Geometry: final body of the model. Coordinates: model frame, mm. A direction names the side the tool comes from. Give positions to 0.01 mm unless a question says otherwise; leave off trailing zeros. Loops run counter-clockwise (first coordinate to the right, second up) from the corner with the lowest first, then second, coordinate; pieces in that order, holes last. Notation, with made-up numbers: (64, -9.75) -> (95, -9.75) arc R16 ccw to (95, 6.25) -> close; hole circle Ø6 at (9, 68.5). An arc over 180 degrees is marked (long way). Answer in a Markdown table with one row per item. Add a question column.
1) Section query B-B (z = -25.5). Return the cut outline in (x, y).
2) Section query D-D (z = 6). Return the cut outline in (x, y).
3) Line query: line 1 (Z direction, x = -75.5, y = 2.65); line 2 (Z direction, x = 78, y = 1); line 3 (X direction, y = 1.4, z = -11.44). Output: solid intervals per line, ascending. Write a range as from..to.
4) Section query C-C (z = 40.5). Return the cut outline in (x, y).
5) First-contact query: P1, Ø5.5, axis at x = 36.3, z = -17.66, coming from the +Y side; P2, Ø5.5, axis at x = -42.5, y = 23, coming from the -Z side; P3, Ø6, axis at y = 23, z = -12.5, coming from the +X side; P4, Ø6, axis at y = 37, z = -21.5, coming from the -X side. Flat tips, straight axial feed; report the tip coordinate or a pass-through.
6) Draft query along X for faces 1 (the flat face through (-37, 31, 38)), 2 (the cylindrical face through (1.17, 2.958, -38.883)), 3 (the flat face through (-51.813, 67.383, 34.158)). Return one class per face: +X half, -X half, draft (parallel to the pull), parting line (faces both ways), or undercut.
7) Section query A-A (x = 0.5). Return the cut outline in (y, z), plus the area to 3 significant figures.
8) Access query for faces 4 (the flat face through (-43.208, 61.647, 34.158)), 5 (the flat face through (-45.56, 37.2, 10.89)), 6 (the flat face through (-37, 31, -17)). Directions: +Z, -Z, +X, -X, +Y, -Y. A direction counts if a zero-diameter tool reaches every point of the face in a straight line with its end or side. Return the directions, or none.
```python
from build123d import *

# Parameters (mm, degrees)
SKETCH1_W                = 170
SKETCH1_H                = 100
BOSS_EXTRUDE1_DEPTH      = 6
BOSS_EXTRUDE2_DEPTH      = 38
BOSS_EXTRUDE2_DEPTH_BACK = 17
SKETCH3_W                = 7.4
SKETCH3_H                = 4
BOSS_EXTRUDE3_DEPTH      = 20
SKETCH5_R                = 1.45
CUT_EXTRUDE1_DEPTH       = 10
SKETCH6_R                = 1.75
CUT_EXTRUDE2_DEPTH       = 20
SKETCH7_R                = 1.65
CUT_EXTRUDE3_DEPTH       = 10
SKETCH9_R                = 1.65
CUT_EXTRUDE6_DEPTH       = 6


with BuildPart() as part:
    # Sketch1 → Boss-Extrude1 (new body)
    with BuildSketch(Plane(origin=(0, 0, 0), x_dir=(1, 0, 0), z_dir=(0, 1, 0))):
        Rectangle(SKETCH1_W, SKETCH1_H)
    extrude(amount=BOSS_EXTRUDE1_DEPTH)

    # Sketch2 → Boss-Extrude2 (add, two sides)
    with BuildSketch(Plane.XY) as boss_extrude2_sk:
        Polygon((-29.617343581, 68.757920077), (-29.617343581, 6), (-48.010328849, 6), (-48.010328849, 38.210127837), (-43.038774216, 36.163017106), align=None)
    extrude(amount=BOSS_EXTRUDE2_DEPTH)
    extrude(boss_extrude2_sk.sketch, amount=-BOSS_EXTRUDE2_DEPTH_BACK)

    # Sketch3 → Boss-Extrude3 (add)
    with BuildSketch(Plane(origin=(-49.531375101, 20.3952721, 0), x_dir=(0, 0, 1), z_dir=(-0.924678098, 0.380749805, 0))):
        with Locations((34.210001, 42.552144992)):
            Rectangle(SKETCH3_W, SKETCH3_H)
        with Locations((-13.189999, 42.552144992)):
            Rectangle(SKETCH3_W, SKETCH3_H)
    extrude(amount=BOSS_EXTRUDE3_DEPTH)

    # Sketch5 → Cut-Extrude1 (cut)
    with BuildSketch(Plane(origin=(15.440221308, 37.49768032, 0), x_dir=(0.924678098, -0.380749805, 0), z_dir=(-0.380749805, -0.924678098, 0))):
        with Locations((-68.566073623, -13.989999)):
            Circle(SKETCH5_R)
        with Locations((-68.566073623, 35.010001)):
            Circle(SKETCH5_R)
        with Locations((-58.566073623, 35.010001)):
            Circle(SKETCH5_R)
        with Locations((-58.566073623, -13.989999)):
            Circle(SKETCH5_R)
    extrude(amount=-CUT_EXTRUDE1_DEPTH, mode=Mode.SUBTRACT)

    # Sketch6 → Cut-Extrude2 (cut)
    with BuildSketch(Plane(origin=(145.967078426, 0, -60.767513946), x_dir=(0, 0, 1), z_dir=(0, -1, 0))):
        with Locations((35.267513946, 221.467078426)):
            Circle(SKETCH6_R)
        with Locations((86.267513946, 221.467078426)):
            Circle(SKETCH6_R)
        with Locations((101.267513946, 145.467078426)):
            Circle(SKETCH6_R)
        with Locations((20.267513946, 145.467078426)):
            Circle(SKETCH6_R)
        with Locations((35.267513946, 70.467078426)):
            Circle(SKETCH6_R)
        with Locations((86.267513946, 70.467078426)):
            Circle(SKETCH6_R)
    extrude(amount=-CUT_EXTRUDE2_DEPTH, mode=Mode.SUBTRACT)

    # Sketch7 → Cut-Extrude3 (cut)
    with BuildSketch(Plane(origin=(0, 6, 0), x_dir=(1, 0, 0), z_dir=(0, 1, 0))):
        with Locations((36.298055455, -30.335990453)):
            Circle(SKETCH7_R)
        with Locations((36.298055455, 17.664009547)):
            Circle(SKETCH7_R)
        with Locations((-21.701944545, 17.664009547)):
            Circle(SKETCH7_R)
        with Locations((-21.701944545, -30.335990453)):
            Circle(SKETCH7_R)
    extrude(amount=-CUT_EXTRUDE3_DEPTH, mode=Mode.SUBTRACT)

    # Sketch9 → Cut-Extrude6 (cut)
    with BuildSketch(Plane(origin=(0, 6, 0), x_dir=(1, 0, 0), z_dir=(0, 1, 0))):
        with Locations((78.25, -11.34)):
            Circle(SKETCH9_R)
        with Locations((78.25, 1.76)):
            Circle(SKETCH9_R)
        with Locations((78.25, 11.44)):
            Circle(SKETCH9_R)
        with Locations((78.25, -1.66)):
            Circle(SKETCH9_R)
    extrude(amount=-CUT_EXTRUDE6_DEPTH, mode=Mode.SUBTRACT)


solid = part.part
```
Evaluation:
| question | item | result |
|---|---|---|
| 1 | outline | (-85, 0) -> (-77.25, 0) -> (-77.25, 6) -> (-85, 6) -> close; (-73.75, 0) -> (73.75, 0) -> (73.75, 6) -> (-73.75, 6) -> close; (77.25, 0) -> (85, 0) -> (85, 6) -> (77.25, 6) -> close |
| 2 | outline | (-85, 0) -> (85, 0) -> (85, 6) -> (-29.62, 6) -> (-29.62, 68.76) -> (-43.04, 36.16) -> (-48.01, 38.21) -> (-48.01, 6) -> (-85, 6) -> close |
| 3 | line 1 | -50..-27.25, -23.75..23.75, 27.25..50 |
| 3 | line 2 | -50..-13.07, -9.81..-3.39, -0.13..0.03, 3.29..9.71, 12.97..50 |
| 3 | line 3 | -85..76.6, 79.9..85 |
| 4 | outline | (-85, 0) -> (-1.25, 0) -> (-1.25, 6) -> (-85, 6) -> close; (2.25, 0) -> (85, 0) -> (85, 6) -> (2.25, 6) -> close |
| 5 | P1 | y = 6 |
| 5 | P2 | z = -17 |
| 5 | P3 | x = -29.62 |
| 5 | P4 | through |
| 6 | face 1 | draft |
| 6 | face 2 | undercut |
| 6 | face 3 | -X half |
| 7 | outline | (0, -50) -> (6, -50) -> (6, -42.25) -> (0, -42.25) -> close; (0, -38.75) -> (6, -38.75) -> (6, 38.75) -> (0, 38.75) -> close; (0, 42.25) -> (6, 42.25) -> (6, 50) -> (0, 50) -> close |
| 7 | area | 558 mm² |
| 8 | face 4 | +Z, -Z, -X |
| 8 | face 5 | +Z, -Z |
| 8 | face 6 | -Z, +X, -X, +Y |
